Input: part model. Units: mm. Frame: model coordinates. Face numbers are marked on the shaded views. A direction names the side the tool comes from. Coordinates: 2 decimals unless noted, no trailing zeros. Loops run counter-clockwise (first coordinate to the right, second up) from the corner with the lowest first, then second, coordinate; pieces in that order, holes last. Notation, with made-up numbers: (15, 68.5) -> (19, 68.5) arc R6 ccw to (19, 72.5) -> close; hole circle Ø1 at (-22, 82.25). An arc over 180 degrees is marked (long way). Put each result on its own line as item: value. Start each with the question number.
1) Set-up query: the marked faces 4 and 5. Return all of +Z, -Z, +X, -X, +Y, -Y with unobstructed straight access to the full face (end or side cutting, diameter ignored); none if empty.
2) Cut plane B-B (x = -16). Return the cut outline in (y, z).
3) Cut plane C-C (y = 25). Return the cut outline in (x, z).
4) Cut plane A-A (z = -16). Return the cut outline in (x, y).
5) Contact query for flat-ended pins moving along their axis: P1, Ø10, axis at x = -10, y = 30.5, coming from the -Z side; P2, Ø17.5, axis at y = 20.5, z = -11, coming from the -X side. Output: stop coordinate, or through.
6) Pull-direction query (X, two-part tool) for the marked faces 1, 2 and 3; classes: pulls with the +X half, pulls with the -X half, needs draft (parallel to the pull), parting line crosses it, or undercut.
7) Cut plane D-D (x = -9.5). Return the cut outline in (y, z).
8) Material intervals for L1, parallel to X at y = 36.5, z = 5; L2, parallel to X at y = 3, z = -15.75, sorted ascending.
Autodesk Inventor part; units mm, degrees
ref_plane "YZ Plane" through (0, 0, 0) normal (1, 0, 0) x (0, 1, 0)
ref_plane "XZ Plane" through (0, 0, 0) normal (0, 1, 0) x (-1, 0, 0)
ref_plane "XY Plane" through (0, 0, 0) normal (0, 0, 1) x (1, 0, 0)
sketch "Sketch2" plane through (0, 0, 0) normal (0, 1, 0) x (-1, 0, 0)
  line L0 (-10, 10) -> (20, 10)
  line L1 (20, 10) -> (20, 0)
  line L2 (0, -20) -> (-10, -20)
  line L3 (-10, -20) -> (-10, 10)
  line L4 (0, 0) -> (20, 0)
  line L5 (20, 0) -> (20, -20)
  line L6 (20, -20) -> (0, -20)
  line L7 (0, -20) -> (0, 0)
  point P0 (5, 0)
  point P1 (0, -5)
  dimension "d4" = 30
  dimension "d5" = 30
  dimension "d6" = 20
  dimension "d7" = 20
extrude "Extrusion2" add sketch "Sketch2" along normal blind 50 contours L0 L1 L4 L7 L2 L3
sketch "Sketch3" plane through (0, 50, 0) normal (0, 1, 0) x (1, 0, 0)
  line L0 (10, 20) -> (0, 20)
  line L1 (0, 20) -> (0, 0)
  line L2 (-20, 0) -> (-20, -10)
  line L3 (-20, -10) -> (10, -10)
  point P0 (-16, -5)
  point P1 (5, 16)
  point P2 (-20, -5)
  point P3 (10, -10)
  point P4 (0, 5)
  dimension "d17" = 4
  dimension "d18" = 5
  dimension "d19" = 4
  dimension "d20" = 5
hole "Hole1" at (-16, 50, 5) at (5, 50, -16) direction (0, -1, 0) diameter 5 end through all
fillet "Fillet1" radius 2 2 edges at (10, 25, 10) (0, 25, 0)
fillet "Fillet2" radius 2 4 edges at (10, 25, -20) (0, 25, -20) (-20, 25, 0) (-20, 25, 10)
properties part number "Base_3D Printed Beam" material "ABS Plastic"
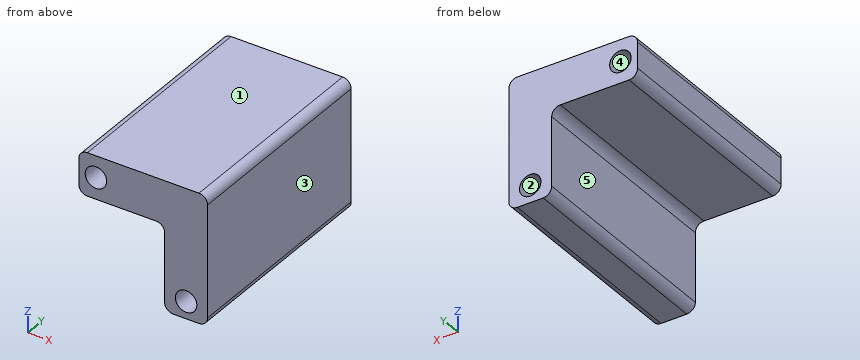
Results found:
1. face 4: +Y, -Y
1. face 5: -Z, -X, +Y, -Y
2. outline: (0, 0) -> (50, 0) -> (50, 2.5) -> (0, 2.5) -> close; (0, 7.5) -> (50, 7.5) -> (50, 10) -> (0, 10) -> close
3. outline: (-20, 2) arc R2 ccw to (-18, 0) -> (-2, 0) arc R2 cw to (0, -2) -> (0, -18) arc R2 ccw to (2, -20) -> (8, -20) arc R2 ccw to (10, -18) -> (10, 8) arc R2 ccw to (8, 10) -> (-18, 10) arc R2 ccw to (-20, 8) -> close; hole circle Ø5 at (-16, 5); hole circle Ø5 at (5, -16)
4. outline: (0, 0) -> (2.5, 0) -> (2.5, 50) -> (0, 50) -> close; (7.5, 0) -> (10, 0) -> (10, 50) -> (7.5, 50) -> close
5. P1: stops at z = 0
5. P2: stops at x = 0
6. face 1: needs draft
6. face 2: undercut
6. face 3: pulls with the +X half
7. outline: (0, 0) -> (50, 0) -> (50, 10) -> (0, 10) -> close
8. L1: x = -20 to -18.5, -13.5 to 10
8. L2: x = 0 to 2.51, 7.49 to 10
